Source: CAD feature listing. Evaluate the final solid. Frame: model axes, mm. Face numbers are marked on the shaded views. A direction names the side the tool comes from. Round coordinates to 2 decimals unless told otherwise and drop trailing zeros. Write each loop counter-clockwise with the first axis right and the second up, starting at its lowest first coordinate (ties: lowest second). Pieces come first, ordered by that corner, then holes.
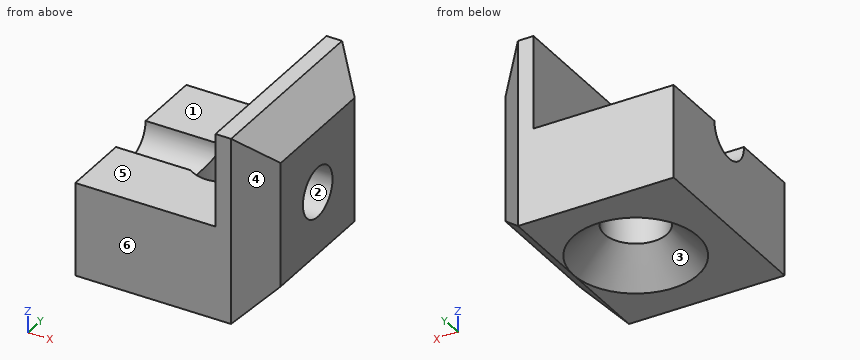
```python
from build123d import *

# Parameters (mm, degrees)
F0_W     = 30
F0_H     = 30
F1_DEPTH = 30
F2_R     = 4
F3_DEPTH = 30.001
F4_R     = 5
F5_DEPTH = 30.001
F6_W     = 30
F6_H     = 15
F7_DEPTH = 22.5
F8_SIZE  = 5
F9_SIZE  = 4.99999


# Not quite as in the source:
# - a fillet or chamfer is up to 0.001 mm smaller than in the source, because OpenCascade refuses the exact size


with BuildPart() as f1:
    # F0 (on Top) → F1 (new body)
    with BuildSketch(Plane.XY):
        with Locations((0.4279911518, -7.855784721)):
            Rectangle(F0_W, F0_H)
    extrude(amount=F1_DEPTH)

    # F2 (on face) → F3 (cut, through all)
    with BuildSketch(Plane(origin=(-14.5720088482, 0, 0), x_dir=(0, -1, 0), z_dir=(-1, 0, 0))):
        with Locations((7.855784721, 15)):
            Circle(F2_R)
    extrude(amount=-F3_DEPTH, mode=Mode.SUBTRACT)

    # F4 (on face) → F5 (cut, through all)
    with BuildSketch(Plane.XY.offset(30)):
        with Locations((0.4279911518, -7.855784721)):
            Circle(F4_R)
    extrude(amount=-F5_DEPTH, mode=Mode.SUBTRACT)

    # F6 (on face) → F7 (cut)
    with BuildSketch(Plane(origin=(-14.5720088482, 0, 0), x_dir=(0, -1, 0), z_dir=(-1, 0, 0))):
        with Locations((7.855784721, 22.5)):
            Rectangle(F6_W, F6_H)
    extrude(amount=-F7_DEPTH, mode=Mode.SUBTRACT)

    # F8
    f8_edges = [f1.edges().sort_by_distance(p)[0] for p in [
        (-4.572009, -7.855785, 0),
    ]]
    chamfer(f8_edges, length=F8_SIZE)

    # F9 (size 5 in the source; OpenCascade refuses exactly that, so slightly less here)
    f9_edges = [f1.edges().sort_by_distance(p)[0] for p in [
        (15.427991, -7.855785, 30),
        (15.427991, -22.855785, 15),
        (15.427991, 7.144215, 15),
        (15.427991, -7.855785, 0),
    ]]
    chamfer(f9_edges, length=F9_SIZE)


solid = f1.part
```
Q1. Section query B-B, the plane y = 3. Output: boundary loops of the cut face in (x, z), and give its area (3 significant figures).
Q2. Mould query, pull axis Z, two halves, no side actions, for the marked faces 1, 2, 3 and 4. Classes: pulls with the +Z half, pulls with the -Z half, needs draft (parallel to the pull), parting line crosses it, or undercut.
Q3. Set-up query: the marked faces 5 and 6. Return all of +Z, -Z, +X, -X, +Y, -Y with unobstructed straight access to the full face (end or side cutting, diameter ignored); none if empty.
Q4. Section query A-A, the plane z = 10. Output: boundary loops of the cut face in (x, y), and give its area (3 significant figures).
Q5. Line query: line 1 (X direction, y = -2, z = 18); line 2 (Z direction, x = -13, y = -22); line 3 (Z direction, x = 8.5, y = -11). Output: solid intervals per line, ascending.
Q6. Section query C-C, the plane y = -4.5. Give the number of separate pieces and of enclosed holes in the cut face, and give its area (3 significant figures).
Q7. Pin query (flat end, axial travel): P1, Ø8, axis at x = 1.5, y = -10, coming from the +Z side; P2, Ø8, axis at y = -5, z = 20, coming from the -X side; P3, Ø2, axis at x = 10.5, z = 23, coming from the +Y side; P4, Ø1.5, axis at x = 11.5, y = -20, coming from the -Z side. Return the tip coordinate at first contact, or that it passes through.
Filled in:
1. outline: (-14.57, 0) - (10.43, 0) - (14.57, 4.14) - (14.57, 25.86) - (10.43, 30) - (7.93, 30) - (7.93, 15) - (-14.57, 15) - close
1. area: 520 mm2
2. face 1: pulls with the +Z half
2. face 2: undercut
2. face 3: pulls with the -Z half
2. face 4: needs draft
3. face 5: +Z, -X, +Y, -Y
3. face 6: +Z, -Z, +X, -X, -Y
4. outline: (-14.57, -22.86) - (10.43, -22.86) - (15.43, -17.86) - (15.43, 2.14) - (10.43, 7.14) - (-14.57, 7.14) - close; hole circle Ø10 at (0.43, -7.86)
4. area: 796 mm2
5. line 1: x = 7.93 to 15.43
5. line 2: z = 0 to 15
5. line 3: z = 1.34 to 12.53, 17.47 to 30
6. separate pieces: 3
6. enclosed holes: 0
6. area: 331 mm2
7. P1: stops at z = 15
7. P2: stops at x = 7.93
7. P3: stops at y = 7.14
7. P4: stops at z = 0.32
